Geometry check sheet. Reference: the model listing, model coordinates, mm. A direction names the side the tool comes from. Give positions to 0.01 mm unless a question says otherwise; leave off trailing zeros. Loops run counter-clockwise (first coordinate to the right, second up) from the corner with the lowest first, then second, coordinate; pieces in that order, holes last. Notation, with made-up numbers: (69.5, 75.25) -> (95.5, 75.25) arc R18 ccw to (95.5, 96.25) -> close; hole circle Ø6 at (-36, -34). An arc over 180 degrees is marked (long way). Answer as a JSON object with one key per item and string values.
Autodesk Inventor part; units mm, degrees
ref_plane "Plano inicial" through (0, 0, 25.4) normal (0, 0, 1) x (1, 0, 0)
ref_plane "Plano final" through (0, 0, 774.6) normal (0, 0, 1) x (1, 0, 0)
ref_plane "Plano de trabajo4" through (19.05, 0, 25.4) normal (0, 0, -1) x (-1, 0, 0)
ref_plane "Plano inicial" through (0, 0, 25.4) normal (0, 0, 1) x (1, 0, 0)
ref_plane "Plano final" through (0, 0, 774.6) normal (0, 0, 1) x (1, 0, 0)
sketch "Boceto" plane through (0, 0, 0) normal (0, 0, 1) x (1, 0, 0)
  line L0 (-25.4, -19.05) -> (-25.4, 19.05)
  line L1 (-19.05, 25.4) -> (19.05, 25.4)
  line L2 (25.4, 19.05) -> (25.4, -19.05)
  line L3 (19.05, -25.4) -> (-19.05, -25.4)
  arc A0 (-25.4, -19.05) -> (-19.05, -25.4) centre (-19.05, -19.05) ccw
  arc A1 (-19.05, 25.4) -> (-25.4, 19.05) centre (-19.05, 19.05) ccw
  arc A2 (25.4, 19.05) -> (19.05, 25.4) centre (19.05, 19.05) ccw
  arc A3 (19.05, -25.4) -> (25.4, -19.05) centre (19.05, -19.05) ccw
  arc A4 (-19.05, 22.225) -> (-22.225, 19.05) centre (-19.05, 19.05) ccw
  line L4 (-19.05, 22.225) -> (19.05, 22.225)
  arc A5 (22.225, 19.05) -> (19.05, 22.225) centre (19.05, 19.05) ccw
  line L5 (22.225, 19.05) -> (22.225, -19.05)
  arc A6 (19.05, -22.225) -> (22.225, -19.05) centre (19.05, -19.05) ccw
  line L6 (19.05, -22.225) -> (-19.05, -22.225)
  arc A7 (-22.225, -19.05) -> (-19.05, -22.225) centre (-19.05, -19.05) ccw
  line L7 (-22.225, -19.05) -> (-22.225, 19.05)
  line L8 (0, 37.4012) -> (0, -37.4012) construction
  line L9 (-37.4012, 0) -> (37.4012, 0) construction
  dimension "d10" = 50.8
  dimension "d11" = 50.8
  dimension "d12" = 3.175
  dimension "d15" = 25.4
  dimension "d16" = 25.4
  dimension "d17" = 6.35
extrude "Cuerpo" add sketch "Boceto" along normal up to surface (749.2 mm away) from surface at 25.4
sketch "Sketch3" plane through (0, 0, 0) normal (0, 0, 1) x (1, 0, 0)
  line L0 (0, 0) -> (10, 0)
ref_plane "Work Plane3" through (0, 0, 0) normal (0, -1, 0) x (1, 0, 0)
ref_plane "Plano de trabajo4" through (19.05, 0, 25.4) normal (0, 0, -1) x (-1, 0, 0)
split "Dividir1" plane through (19.05, 0, 25.4) removes the side toward (0, 0, -1)
ref_plane "Plano de trabajo5" through (19.05, 400, 774.6) normal (0, 0, 1) x (1, 0, 0)
split "Dividir2" plane through (19.05, 400, 774.6) removes the side toward (0, 0, 1)
sketch "Sketch4" plane through (0, 0, 0) normal (0, -1, 0) x (1, 0, 0)
  line L0 (-2, 25.4) -> (12, 25.4)
  line L1 (-2, 774.6) -> (12, 774.6)
  dimension "d19" = 749.2
equation "\"d10\" = G_H"
equation "\"d11\" = G_W"
equation "\"d12\" = G_T"
equation "\"d15\" = 0.5 * d10"
equation "\"d16\" = 0.5 * d11"
equation "\"d17\" = G_IR"
equation "\"d3\" = G_L"
equation "\"G_W\" = 50.8"
equation "\"G_H\" = 50.8"
equation "\"G_T\" = 3.175"
equation "\"G_IR\" = 6.35"
equation "\"G_L\" = d19"
equation "\"G_OFFSET_START\" = -25.4"
equation "\"G_OFFSET_END\" = -25.4"
equation "\"d13\" = -G_OFFSET_START"
equation "\"d14\" = G_OFFSET_END + B_L"
equation "\"B_L\" = 800"
properties part number "AISC - 2 x 2 x 1/8 - 29,496" material "Acero, suave"
1) Tool access check on faces 1 (the face through (-0.1, -22.5, 25.4)), 2 (the face through (0, -22.225, 395)). Record the directions out of +Z, -Z, +X, -X, +Y, -Y that give a thin tool (end or side, any length) a straight path to the whole face; none if there is none.
Geometry check:
{"face 1": "-Z, +X, -X, +Y, -Y", "face 2": "+Z, -Z"}
2) Section check B-B on y = 2.5. Record the cut outline in (x, z) (3 decimals), plus the area to 3 significant figures.
Geometry check:
{"outline": "(-25.4, 25.4) -> (-22.225, 25.4) -> (-22.225, 774.6) -> (-25.4, 774.6) -> close; (22.225, 25.4) -> (25.4, 25.4) -> (25.4, 774.6) -> (22.225, 774.6) -> close", "area": "4,760 mm2"}
3) Section check A-A on z = 712. Record the cut outline in (x, y) (3 decimals), plus the area to 3 significant figures.
Geometry check:
{"outline": "(-25.4, -19.05) arc R6.35 ccw to (-19.05, -25.4) -> (19.05, -25.4) arc R6.35 ccw to (25.4, -19.05) -> (25.4, 19.05) arc R6.35 ccw to (19.05, 25.4) -> (-19.05, 25.4) arc R6.35 ccw to (-25.4, 19.05) -> close; hole (-22.225, -19.05) arc R3.175 ccw to (-19.05, -22.225) -> (19.05, -22.225) arc R3.175 ccw to (22.225, -19.05) -> (22.225, 19.05) arc R3.175 ccw to (19.05, 22.225) -> (-19.05, 22.225) arc R3.175 ccw to (-22.225, 19.05) -> close", "area": "579 mm2"}
4) Material ranges on line 1 along Y through (x, z) = (-18, 65.5) (3 decimals); line 2 along Y through (x, z) = (21, 536), recorded low to high. Write a range as from..to.
Geometry check:
{"line 1": "y = -25.4..-22.225, 22.225..25.4", "line 2": "y = -25.09..-21.56, 21.56..25.09"}
5) Draft check along X on faces 3 (the face through (25.4, 0, 395)), 4 (the face through (22.225, 0, 395)), 5 (the face through (0, 22.225, 395)), 6 (the face through (0, 25.4, 395)). Enter one of: pulls with the +X half, pulls with the -X half, needs draft (parallel to the pull), parting line crosses it, or undercut.
Geometry check:
{"face 3": "pulls with the +X half", "face 4": "undercut", "face 5": "undercut", "face 6": "needs draft"}
